from build123d import *

# Parameters (mm, degrees)
EXTRUDE_THIN1_DEPTH = 1365.25
FILLET1_R           = 1.27


with BuildPart() as part:
    # Sketch1 → Extrude-Thin1 (new body)
    with BuildSketch(Plane.XY):
        with BuildLine():
            Line((0, 0), (-22.225, 0))
            Line((-22.225, 0), (-22.225, 19.05))
            ThreePointArc((-22.225, 19.05), (-19.418669962, 20.212419962), (-18.25625, 23.01875))
            Line((-18.25625, 23.01875), (-18.25625, 79.375))
            ThreePointArc((-18.25625, 79.375), (-19.418669962, 82.181330038), (-22.225, 83.34375))
            Line((-22.225, 83.34375), (-22.225, 86.51875))
            Line((-22.225, 86.51875), (-24.765, 86.51875))
            ThreePointArc((-24.765, 86.51875), (-27.14625, 88.9), (-24.765, 91.28125))
            Line((-24.765, 91.28125), (-22.225, 91.28125))
            Line((-22.225, 91.28125), (-22.225, 94.45625))
            ThreePointArc((-22.225, 94.45625), (-30.157584675, 102.15609622), (-32.478342254, 112.964778641))
            ThreePointArc((-32.478342254, 112.964778641), (-30.377697482, 116.671337824), (-26.19375, 117.475))
            Line((-26.19375, 117.475), (-26.19375, 120.65))
            Line((-26.19375, 120.65), (-32.54375, 120.65))
            Line((-32.54375, 120.65), (-32.54375, 136.525))
            Line((-32.54375, 136.525), (0, 136.525))
            Line((0, 136.525), (0, 135.255))
            Line((0, 135.255), (-31.27375, 135.255))
            Line((-31.27375, 135.255), (-31.27375, 121.92))
            Line((-31.27375, 121.92), (-24.92375, 121.92))
            Line((-24.92375, 121.92), (-24.92375, 115.426165066))
            ThreePointArc((-24.92375, 115.426165066), (-28.855388092, 116.071729842), (-31.21270277, 112.859627808))
            ThreePointArc((-31.21270277, 112.859627808), (-28.857537425, 102.438637116), (-20.955, 95.248800326))
            Line((-20.955, 95.248800326), (-20.955, 90.01125))
            Line((-20.955, 90.01125), (-24.765, 90.01125))
            ThreePointArc((-24.765, 90.01125), (-25.87625, 88.9), (-24.765, 87.78875))
            Line((-24.765, 87.78875), (-20.955, 87.78875))
            Line((-20.955, 87.78875), (-20.955, 84.457479863))
            ThreePointArc((-20.955, 84.457479863), (-18.09597384, 82.599227742), (-16.98625, 79.375))
            Line((-16.98625, 79.375), (-16.98625, 23.01875))
            ThreePointArc((-16.98625, 23.01875), (-18.09597384, 19.794522258), (-20.955, 17.936270137))
            Line((-20.955, 17.936270137), (-20.955, 1.27))
            Line((-20.955, 1.27), (0, 1.27))
            Line((0, 1.27), (0, 0))
        make_face()
    extrude(amount=-EXTRUDE_THIN1_DEPTH)

    # Fillet1
    fillet1_edges = [part.edges().sort_by_distance(p)[0] for p in [
        (-24.92375, 121.92, -682.625),
        (-24.92375, 115.426165066, -682.625),
        (-20.955, 95.248800326, -682.625),
        (-20.955, 90.01125, -682.625),
        (-20.955, 87.78875, -682.625),
        (-22.225, 0, -682.625),
        (-22.225, 19.05, -682.625),
        (-22.225, 83.34375, -682.625),
        (-32.54375, 120.65, -682.625),
        (-32.54375, 136.525, -682.625),
    ]]
    fillet(fillet1_edges, radius=FILLET1_R)


solid = part.part
Part model, mm, in its own coordinate system. A direction names the side the tool comes from. Round coordinates to 2 decimals unless told otherwise and drop trailing zeros. Loops run counter-clockwise (first coordinate to the right, second up) from the corner with the lowest first, then second, coordinate; pieces in that order, holes last. Notation, with made-up numbers: (-18, 34.5) - (16, 34.5) arc R20 ccw to (16, 61.5) - close; hole circle Ø11 at (17.5, 69.25). An arc over 180 degrees is marked (long way). Answer as a JSON object with one key per item and string values.
Item 1: Wall check: L1, parallel to Y at x = -12.5, z = -869 (3 decimals); L2, parallel to X at y = 35.5, z = -1294; L3, parallel to X at y = 92.5, z = -749.5 (3 decimals). Give the ranges that are in metal, low to high.
Output:
{"L1": "0 to 1.27, 135.255 to 136.525", "L2": "-18.26 to -16.99", "L3": "-22.225 to -20.955"}
Item 2: Tool access for faces 1 (the face through (-11, 1.27, -673)), 2 (the face through (-10, 0, -673)): list every direction of +Z, -Z, +X, -X, +Y, -Y with a clear straight run to the whole face (end or side of a thin tool).
Output:
{"face 1": "+Z, -Z, +X", "face 2": "+Z, -Z, +X, -X, -Y"}
Item 3: Pull direction Y, two halves, no side cores. Call faces 3 (the face through (-17.4, 63.5, -1365.25)), 4 (the face through (-16, 136.525, -673)), 5 (the face through (-16.986, 52, -673)), 6 (the face through (-18.256, 51, -673)): pulls with the +Y half, pulls with the -Y half, needs draft (parallel to the pull), parting line crosses it, or undercut.
Output:
{"face 3": "needs draft", "face 4": "pulls with the +Y half", "face 5": "undercut", "face 6": "undercut"}
Item 4: Band-saw the part on A-A on y = 48. List the corners of the cut face in (x, z), plus the area to 3 significant figures.
Output:
{"outline": "(-18.26, -1365.25) - (-16.99, -1365.25) - (-16.99, 0) - (-18.26, 0) - close", "area": "1,730 mm2"}
Item 5: Pin check, flat tips, straight feed: pin 1 (2.5 mm diameter, centred on y = 92, z = -1000.5, fed in from -X); pin 2 (1 mm diameter, centred on y = 84, z = -457.5, fed in from +X); pin 3 (18.5 mm diameter, centred on y = 8.5, z = -686.5, fed in from -X) (3 decimals). Stop position of each tip, or through.
Output:
{"pin 1": "x = -26.26", "pin 2": "x = -19", "pin 3": "x = -22.225"}
